Input: part model. Units: mm. Frame: model coordinates. Round coordinates to 2 decimals unless told otherwise and drop trailing zeros. Order: outer loops, then holes, each group sorted by start corner. A loop starts at its lowest first (then second) coordinate and runs counter-clockwise, first axis right, second up. Notation, with made-up numbers: (-5.75, 62) -> (24.25, 62) arc R19 ccw to (24.25, 93) -> close; hole circle Ø10 at (-38, 89.5). An arc over 180 degrees is marked (long way). Use a Markdown table: item, result.
from build123d import *

# Parameters (mm, degrees)
SKETCH1_W             = 300
SKETCH1_H             = 273
BASE_FLANGE1_DEPTH    = 2
M25_CLEARANCE_HOLE1_D = 27


# Sheet-metal steps are written as plain solids
with BuildPart() as part:
    # Sketch1 → Base-Flange1 (new body)
    with BuildSketch(Plane.XY):
        with Locations((-150, 136.5)):
            Rectangle(SKETCH1_W, SKETCH1_H)
    extrude(amount=-BASE_FLANGE1_DEPTH)

    # Sketch8 → CSK for M3 Oval Head Machine Screw1 (revolve, cut)
    with BuildSketch(Plane(origin=(-293, 249.78, 0), x_dir=(0, -1, 0), z_dir=(1, 0, 0))):
        Polygon((0, 0), (0, 2), (1.6, 2), (1.6, 1.55), (3.15, 0), align=None)
    csk_for_m3_oval_head_machine_screw1 = revolve(axis=Axis((-293, 249.78, 6.35), (0, 0, -1)), mode=Mode.SUBTRACT)

    # Mirror1: CSK for M3 Oval Head Machine Screw1 across plane
    add(csk_for_m3_oval_head_machine_screw1.mirror(Plane.ZY.offset(150)), mode=Mode.SUBTRACT)

    # M25 Clearance Hole1 (through all)
    with Locations(Plane.XY):
        with Locations((-150, 233)):
            Hole(M25_CLEARANCE_HOLE1_D / 2)


solid = part.part
1) Line query: L1, parallel to X at y = 249.78, z = -1.8; L2, parallel to Y at x = -150, z = -0.9; L3, parallel to Y at x = -152, z = -1.4. Output: solid intervals per line, ascending. Write a range as [from, to].
Results found:
| item | result |
|---|---|
| L1 | x = [-300, -294.6], [-291.4, -8.6], [-5.4, 0] |
| L2 | y = [0, 219.5], [246.5, 273] |
| L3 | y = [0, 219.65], [246.35, 273] |
2) Pull-direction query (X, two-part tool) for faces 1 (the cylindrical face through (-156.229, 221.023, -1.014)), 2 (the flat face through (-152, 138, -2)); classes: +X half, -X half, draft (parallel to the pull), parting line (faces both ways), or undercut.
Results found:
| item | result |
|---|---|
| face 1 | undercut |
| face 2 | draft |
3) Cut plane A-A on y = 233. Return loops of the section in (x, z), and give its area (3 significant figures).
Results found:
| item | result |
|---|---|
| outline | (-300, -2) -> (-163.5, -2) -> (-163.5, 0) -> (-300, 0) -> close; (-136.5, -2) -> (0, -2) -> (0, 0) -> (-136.5, 0) -> close |
| area | 546 mm² |
4) Cut plane B-B on x = -150. Return loops of the section in (y, z), and give its area (3 significant figures).
Results found:
| item | result |
|---|---|
| outline | (0, -2) -> (219.5, -2) -> (219.5, 0) -> (0, 0) -> close; (246.5, -2) -> (273, -2) -> (273, 0) -> (246.5, 0) -> close |
| area | 492 mm² |
5) Pin query (flat end, axial travel): pin 1 Ø3 at (x, y) = (-293, 249.78) entering from +Z. Return the tip coordinate at first contact, or that it passes through.
Results found:
| item | result |
|---|---|
| pin 1 | passes through |
